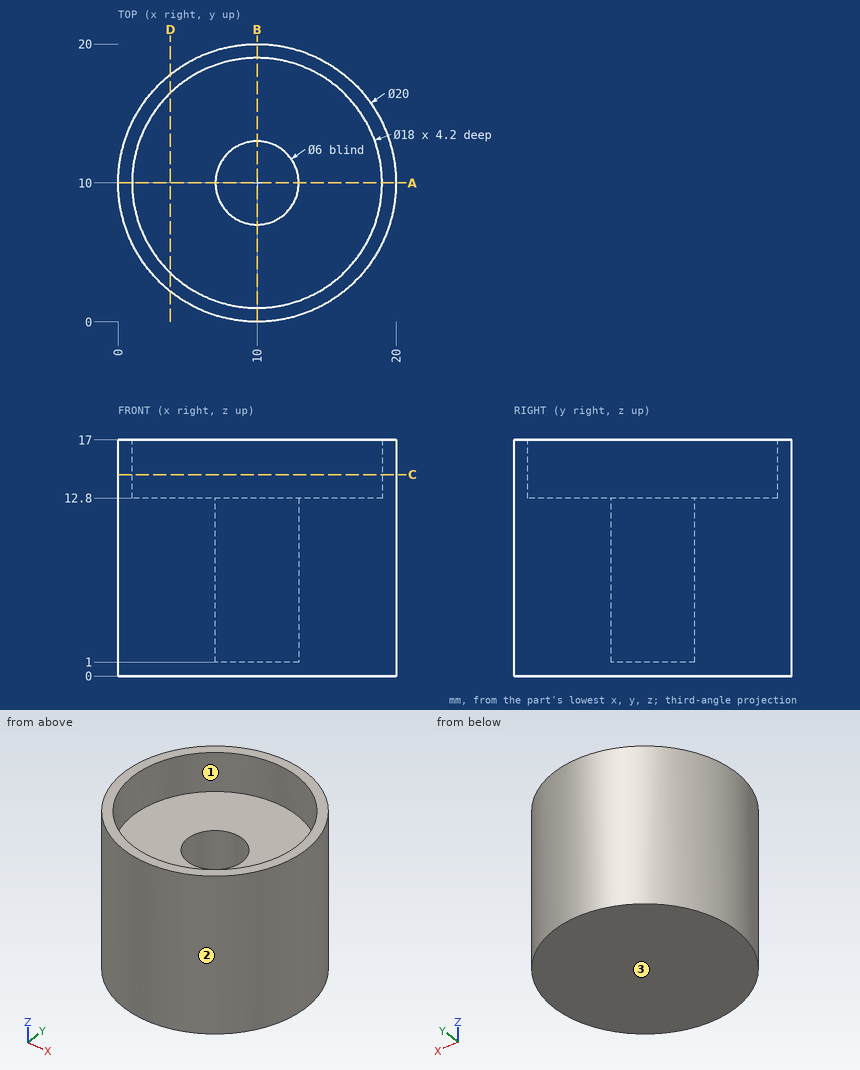
Drawing for the job (mm, zero at the part's lowest x, y, z). Coordinates: 2 decimals unless noted, no trailing zeros. Order: outer loops, then holes, each group sorted by start corner. A loop starts at its lowest first (then second) coordinate and runs counter-clockwise, first axis right, second up.
Item 1: Pin check, flat tips, straight feed: pin 1 Ø8 at (x, y) = (10, 10) entering from +Z; pin 2 Ø11 at (x, y) = (10, 10) entering from -Z; pin 3 Ø1 at (y, z) = (12, 12) entering from +X; pin 4 Ø1.5 at (x, z) = (3, 6.5) entering from +Y. Stop position of each tip, or through.
Check sheet entries:
pin 1: stops at z = 12.8
pin 2: stops at z = 0
pin 3: stops at x = 19.89
pin 4: stops at y = 17.81
Item 2: Drill centre lines: L1, parallel to Y at x = 10, z = 8.5; L2, parallel to Y at x = 10, z = 14.4; L3, parallel to Z at x = 5.75, y = 4.25. Where is each one in solid material? Low to high.
Check sheet entries:
L1: y = 0 to 7, 13 to 20
L2: y = 0 to 1, 19 to 20
L3: z = 0 to 12.8
Item 3: Band-saw the part on D-D on x = 3.75. List the corners of the cut face in (y, z), plus the area to 3 significant figures.
Check sheet entries:
outline: (2.19, 0) - (17.81, 0) - (17.81, 17) - (16.48, 17) - (16.48, 12.8) - (3.52, 12.8) - (3.52, 17) - (2.19, 17) - close
area: 211 mm2
Item 4: Band-saw the part on C-C on z = 14.5. List the corners of the cut face in (x, y).
Check sheet entries:
outline: circle Ø20 at (10, 10); hole circle Ø18 at (10, 10)
Item 5: Band-saw the part on A-A on y = 10. List the corners of the cut face in (x, z), plus the area to 3 significant figures.
Check sheet entries:
outline: (0, 0) - (20, 0) - (20, 17) - (19, 17) - (19, 12.8) - (13, 12.8) - (13, 1) - (7, 1) - (7, 12.8) - (1, 12.8) - (1, 17) - (0, 17) - close
area: 194 mm2
Item 6: Two-plate mould, pull along Y, no slides. Class the marked faces 1, 2 and 3: +Y half, -Y half, draft (parallel to the pull), parting line (faces both ways), or undercut.
Check sheet entries:
face 1: undercut
face 2: parting line
face 3: draft
